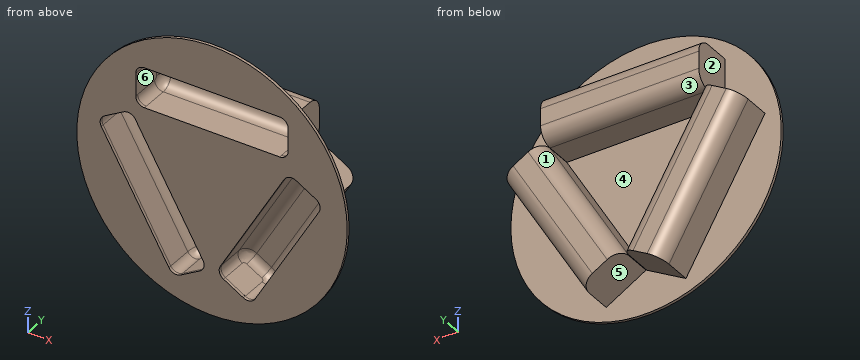
from build123d import *

# Parameters (mm, degrees)
BOSS_EXTRUDE1_DEPTH     = 15
SKETCH1_W               = 55
SKETCH1_H               = 15.959882119
BOSS_EXTRUDE1_2_DEPTH   = 15
BOSS_EXTRUDE1_3_DEPTH   = 15
FILLET1_R               = 5
FILLET2_R               = 5
FILLET3_R               = 5
FILLET4_R               = 5
FILLET5_R               = 5
FILLET6_R               = 5
SHELL1_T                = -1
SHELL2_T                = -1
SHELL3_T                = -1
FILLET7_R               = 3
FILLET8_R               = 3
FILLET9_R               = 3
FILLET10_R              = 3
FILLET11_R              = 3
FILLET12_R              = 3
SKETCH2_R               = 47
BOSS_EXTRUDE2_DEPTH     = 1
CUT_EXTRUDE1_DEPTH      = 1
CUT_EXTRUDE1_DEPTH_BACK = 13


with BuildPart() as part:
    # Sketch1 → Boss-Extrude1 (new body)
    with BuildSketch(Plane(origin=(0, 0, 0), x_dir=(1, 0, 0), z_dir=(0, 1, 0))):
        Polygon((0.023694735, 0.013680161), (13.856406461, 8), (41.356406461, -39.631397208), (27.523694735, -47.617717047), align=None)
    extrude(amount=BOSS_EXTRUDE1_DEPTH)

    # Fillet3
    fillet3_edges = [part.edges().sort_by_distance(p)[0] for p in [
        (27.606406461, 15, 15.815698604),
    ]]
    fillet(fillet3_edges, radius=FILLET3_R)

    # Fillet4
    fillet4_edges = [part.edges().sort_by_distance(p)[0] for p in [
        (13.773694735, 15, 23.802018443),
    ]]
    fillet(fillet4_edges, radius=FILLET4_R)

    # Shell3
    shell3_openings = [part.faces().sort_by_distance(p)[0] for p in [
        (20.690050598, 0, 19.808858523),
    ]]
    offset(amount=SHELL3_T, openings=shell3_openings, kind=Kind.INTERSECTION)

    # Fillet9
    fillet9_edges = [part.edges().sort_by_distance(p)[0] for p in [
        (2.404332011, 12.828427125, -0.233441195),
        (12.475769184, 12.828427125, -6.048188159),
        (13.490381057, 5, -6.633974596),
        (1.389720138, 5, 0.352345242),
        (7.440050598, 14, -3.140814677),
    ]]
    fillet(fillet9_edges, radius=FILLET9_R)

    # Fillet12
    fillet12_edges = [part.edges().sort_by_distance(p)[0] for p in [
        (39.990381057, 5, 39.265371804),
        (28.904332011, 12.828427125, 45.665905205),
        (27.889720138, 5, 46.251691643),
        (38.975769184, 12.828427125, 39.851158242),
        (33.940050598, 14, 42.758531724),
    ]]
    fillet(fillet12_edges, radius=FILLET12_R)



with BuildPart() as body_2:
    # Sketch1 → Boss-Extrude1 2 (new body)
    with BuildSketch(Plane(origin=(0, 0, 0), x_dir=(1, 0, 0), z_dir=(0, 1, 0))):
        with Locations((0, -55.651456149)):
            Rectangle(SKETCH1_W, SKETCH1_H)
    extrude(amount=BOSS_EXTRUDE1_2_DEPTH)

    # Fillet1
    fillet1_edges = [body_2.edges().sort_by_distance(p)[0] for p in [
        (0, 15, 63.631397208),
    ]]
    fillet(fillet1_edges, radius=FILLET1_R)

    # Fillet2
    fillet2_edges = [body_2.edges().sort_by_distance(p)[0] for p in [
        (0, 15, 47.671515089),
    ]]
    fillet(fillet2_edges, radius=FILLET2_R)

    # Shell2
    shell2_openings = [body_2.faces().sort_by_distance(p)[0] for p in [
        (0, 0, 55.651456149),
    ]]
    offset(amount=SHELL2_T, openings=shell2_openings, kind=Kind.INTERSECTION)

    # Fillet10
    fillet10_edges = [body_2.edges().sort_by_distance(p)[0] for p in [
        (-26.5, 5, 62.631397208),
        (-26.5, 12.828427125, 49.843087964),
        (-26.5, 5, 48.671515089),
        (-26.5, 12.828427125, 61.459824333),
        (-26.5, 14, 55.651456149),
    ]]
    fillet(fillet10_edges, radius=FILLET10_R)

    # Fillet11
    fillet11_edges = [body_2.edges().sort_by_distance(p)[0] for p in [
        (26.5, 12.828427125, 49.843087964),
        (26.5, 12.828427125, 61.459824333),
        (26.5, 5, 62.631397208),
        (26.5, 5, 48.671515089),
        (26.5, 14, 55.651456149),
    ]]
    fillet(fillet11_edges, radius=FILLET11_R)


with BuildPart() as body_3:
    # Sketch1 → Boss-Extrude1 3 (new body)
    with BuildSketch(Plane(origin=(0, 0, 0), x_dir=(1, 0, 0), z_dir=(0, 1, 0))):
        Polygon((-27.789098516, -47.464486102), (-41.356406461, -39.631397208), (-13.856406461, 8), (-0.289098516, 0.166911106), align=None)
    extrude(amount=BOSS_EXTRUDE1_3_DEPTH)

    # Fillet5
    fillet5_edges = [body_3.edges().sort_by_distance(p)[0] for p in [
        (-14.039098516, 15, 23.648787498),
    ]]
    fillet(fillet5_edges, radius=FILLET5_R)

    # Fillet6
    fillet6_edges = [body_3.edges().sort_by_distance(p)[0] for p in [
        (-27.606406461, 15, 15.815698604),
    ]]
    fillet(fillet6_edges, radius=FILLET6_R)

    # Shell1
    shell1_openings = [body_3.faces().sort_by_distance(p)[0] for p in [
        (-20.822752488, 0, 19.732243051),
    ]]
    offset(amount=SHELL1_T, openings=shell1_openings, kind=Kind.INTERSECTION)

    # Fillet7
    fillet7_edges = [body_3.edges().sort_by_distance(p)[0] for p in [
        (-28.155123919, 5, 46.098460699),
        (-38.975769184, 12.828427125, 39.851158242),
        (-39.990381057, 5, 39.265371804),
        (-29.169735792, 12.828427125, 45.512674261),
        (-34.072752488, 14, 42.681916251),
    ]]
    fillet(fillet7_edges, radius=FILLET7_R)

    # Fillet8
    fillet8_edges = [body_3.edges().sort_by_distance(p)[0] for p in [
        (-12.475769184, 12.828427125, -6.048188159),
        (-2.669735792, 12.828427125, -0.38667214),
        (-1.655123919, 5, 0.199114298),
        (-13.490381057, 5, -6.633974596),
        (-7.572752488, 14, -3.217430149),
    ]]
    fillet(fillet8_edges, radius=FILLET8_R)


with BuildPart() as part_1:
    add(part.part)

    add(body_2.part)  # Boss-Extrude2 merges body 2

    add(body_3.part)  # Boss-Extrude2 merges body 3
    # Sketch2 → Boss-Extrude2 (add)
    with BuildSketch(Plane(origin=(0, 0, 0), x_dir=(1, 0, 0), z_dir=(0, 1, 0))):
        with Locations((0, -31.745023024)):
            Circle(SKETCH2_R)
    extrude(amount=BOSS_EXTRUDE2_DEPTH)

    # Sketch3 → Cut-Extrude1 (cut, two sides)
    with BuildSketch(Plane(origin=(0, 0, 0), x_dir=(1, 0, 0), z_dir=(0, 1, 0))) as cut_extrude1_sk:
        with BuildLine():
            Line((3.987006883, 1.141166124), (10.886295934, 5.136526307))
            ThreePointArc((10.886295934, 5.136526307), (13.164256292, 5.43870151), (14.98777262, 4.04041633))
            Line((14.98777262, 4.04041633), (37.191342951, -34.417295593))
            ThreePointArc((37.191342951, -34.417295593), (37.491044219, -36.693752728), (36.09326674, -38.515371804))
            Line((36.09326674, -38.515371804), (29.188758244, -42.501691643))
            ThreePointArc((29.188758244, -42.501691643), (26.912301109, -42.801392911), (25.090682033, -41.403615432))
            Line((25.090682033, -41.403615432), (2.892331147, -2.954943853))
            ThreePointArc((2.892331147, -2.954943853), (2.592122178, -0.68038397), (3.987006883, 1.141166124))
        make_face()
        with BuildLine():
            Line((-23.5, -48.671515089), (23.5, -48.671515089))
            ThreePointArc((23.5, -48.671515089), (25.621320344, -49.550194746), (26.5, -51.671515089))
            Line((26.5, -51.671515089), (26.5, -59.631397208))
            ThreePointArc((26.5, -59.631397208), (25.621320344, -61.752717552), (23.5, -62.631397208))
            Line((23.5, -62.631397208), (-23.5, -62.631397208))
            ThreePointArc((-23.5, -62.631397208), (-25.621320344, -61.752717552), (-26.5, -59.631397208))
            Line((-26.5, -59.631397208), (-26.5, -51.671515089))
            ThreePointArc((-26.5, -51.671515089), (-25.621320344, -49.550194746), (-23.5, -48.671515089))
        make_face()
        with BuildLine():
            Line((-26.655123919, -43.500384487), (-3.155123919, -2.797190509))
            ThreePointArc((-3.155123919, -2.797190509), (-2.855422652, -0.520733374), (-4.253200131, 1.300885702))
            Line((-4.253200131, 1.300885702), (-10.892304845, 5.133974596))
            ThreePointArc((-10.892304845, 5.133974596), (-13.168761981, 5.433675864), (-14.990381057, 4.035898385))
            Line((-14.990381057, 4.035898385), (-38.490381057, -36.667295593))
            ThreePointArc((-38.490381057, -36.667295593), (-38.790082324, -38.943752728), (-37.392304845, -40.765371804))
            Line((-37.392304845, -40.765371804), (-30.753200131, -44.598460699))
            ThreePointArc((-30.753200131, -44.598460699), (-28.476742995, -44.898161966), (-26.655123919, -43.500384487))
        make_face()
    extrude(amount=CUT_EXTRUDE1_DEPTH, mode=Mode.SUBTRACT)
    extrude(cut_extrude1_sk.sketch, amount=-CUT_EXTRUDE1_DEPTH_BACK, mode=Mode.SUBTRACT)


solid = part_1.part
The model under review builds one solid part; all positions refer to its coordinate system, in mm. Face numbers are marked on the shaded views. A direction names the side the tool comes from. Give positions to 0.01 mm unless a question says otherwise; leave off trailing zeros. One line per question, with ' | ' between items. Start each with the question number.
1) Wall thickness on L1, parallel to X at y = 7, z = 57.5; L2, parallel to X at y = 4, z = 39; L3, parallel to Z at x = 5, y = 8: over which ranges is each line inside the solid? List them lowest first. Write a range as from..to.
2) Clearance check with flat-ended pins moving along their axes: P1, Ø1, axis at x = -25.5, y = 3, coming from the -Z side; P2, Ø3, axis at x = -15.5, z = 35, coming from the +Y side; P3, Ø1, axis at x = -12, z = 18, coming from the +Y side. State where each tip first meets the part, or that it passes through.
3) Consider section A-A, the plane y = 8. State how many separate pieces and enclosed holes the cut face has, then the cut area to 3 significant figures.
4) For the marked faces 4, 5 and 6, list the 3-axis set-ups (+Z, -Z, +X, -X, +Y, -Y) from which the entire face can be reached by the end or side of a thin tool; tool diameter is ignored.
5) Mouldability with a two-part tool opening along X and no side actions: class the marked faces 1, 2 and 3 as pulls with the +X half, pulls with the -X half, needs draft (parallel to the pull), parting line crosses it, or undercut.
Found:
1) L1: x = -27.5..-26.5, 26.5..27.5 | L2: x = -40.99..-38.77, -24.06..-22.9, 22.55..23.7, 38.77..40.99 | L3: z = -2.89..-1.73, 6.61..8.61, 47.67..48.67, 62.63..63.63
2) P1: stops at z = 11.3 | P2: stops at y = 1 | P3: stops at y = 13.63
3) separate pieces: 3 | enclosed holes: 3 | area: 436 mm²
4) face 4: +Y | face 5: -Z, +Y | face 6: -Y
5) face 1: undercut | face 2: pulls with the -X half | face 3: needs draft
